The model under review builds one solid part; all positions refer to its coordinate system, in mm. A direction names the side the tool comes from. Coordinates: 2 decimals unless noted, no trailing zeros. Write each loop counter-clockwise with the first axis right and the second up, starting at its lowest first coordinate (ties: lowest second). Pieces come first, ordered by that corner, then holes.
1) Add section B-B, the plane z = 1.25. State the section outline as (x, y) points, then the cut area to 3 significant figures.
2) Add section C-C, the plane x = 3.25. Give the number of separate pieces and of enclosed holes in the cut face, then the cut area to 3 significant figures.
3) Mouldability with a two-part tool opening along X and no side actions: class faces 1 (the flat face through (3, 0, 0)), 2 (the flat face through (-3.458, 1.996, 1.014)), 3 (the cylindrical face through (-5.158, 3.955, 0.887)) as released by +X, released by -X, zero draft, split by the parting line, or undercut.
4) Machinability: for faces 4 (the flat face through (3, 0, 2)), 5 (the flat face through (0.5, 4, 1)), which of the approach directions +Z, -Z, +X, -X, +Y, -Y give a long, thin tool a straight path to every point of the face, cutting with its end or side? Answer none if there is none.
5) For line 1 (Y direction, x = -0.75, z = 0.4); line 2 (X direction, y = -3.75, z = 0.45); line 3 (X direction, y = 3, z = 1.9), list the stretches that pass through material, from the lowest coordinate up.
6) Add section A-A, the plane x = 0. State the section outline as (y, z) points.
7) For P1, Ø0.8, axis at y = -4, z = 1, coming from the +X side; P2, Ø4, axis at x = 1.5, y = -4, coming from the +Z side; P3, Ø0.5, axis at y = 3.5, z = 1, coming from the +X side, all flat-tipped, find the tip position at first contact; note any pin that passes through.
Autodesk Inventor part; units mm, degrees
ref_plane "YZ Plane" through (0, 0, 0) normal (1, 0, 0) x (0, 1, 0)
ref_plane "XZ Plane" through (0, 0, 0) normal (0, 1, 0) x (-1, 0, 0)
ref_plane "XY Plane" through (0, 0, 0) normal (0, 0, 1) x (1, 0, 0)
sketch "スケッチ1" plane through (0, 0, 0) normal (0, 0, 1) x (1, 0, 0)
  circle A0 centre (0, 0) radius 6.5
  arc A1 (2, -1.5) -> (-2, -1.5) centre (0, 0) ccw
  line L0 (2, -1.5) -> (-2, -1.5)
  arc A2 (-2, -1.5) -> (2, -1.5) centre (0, 0) ccw
  dimension "d0" = 13
  dimension "d1" = 5
  dimension "d2" = 4
extrude "押し出し1" add sketch "スケッチ1" along normal blind 2 contours A0 | A2 L0
sketch "スケッチ2" plane through (0, 0, 2) normal (0, 0, 1) x (1, 0, 0)
  circle A0 centre (0, 0) radius 6.5
  line L0 (0.5, -6.5) -> (0, -6.5)
  line L1 (0, -6.5) -> (-0.5, -6.5)
  arc A1 (2, -1.5) -> (-2, -1.5) centre (0, 0) ccw
  arc A2 (3.8971, 2.25) -> (0.5, 4.4721) centre (0, 0) ccw
  arc A3 (3.0311, 1.75) -> (0.5, 3.4641) centre (0, 0) ccw
  arc A4 (-0.5, 4.4721) -> (-3.8971, 2.25) centre (0, 0) ccw
  arc A5 (-0.5, 3.4641) -> (-3.0311, 1.75) centre (0, 0) ccw
  arc A6 (0.5, -3.4641) -> (3.0311, -1.75) centre (0, 0) ccw
  arc A7 (-3.0311, -1.75) -> (-0.5, -3.4641) centre (0, 0) ccw
  arc A8 (-3.8971, -2.25) -> (-0.5, -4.4721) centre (0, 0) ccw
  arc A9 (0.5, -4.4721) -> (3.8971, -2.25) centre (0, 0) ccw
  line L2 (-3.0311, 1.75) -> (-3.8971, 2.25)
  line L3 (-0.5, 3.4641) -> (-0.5, 4.4721)
  line L4 (0.5, 4.4721) -> (0.5, 3.4641)
  line L5 (3.0311, 1.75) -> (3.8971, 2.25)
  line L6 (-3.0311, -1.75) -> (-3.8971, -2.25)
  line L7 (3.0311, -1.75) -> (3.8971, -2.25)
  line L8 (-0.5, -4.4721) -> (-0.5, -3.4641)
  line L9 (0.5, -3.4641) -> (0.5, -4.4721)
extrude "押し出し2" cut sketch "スケッチ2" against normal through all contours L5 A3 L4 A2 | L3 A5 L2 A4 | A6 L7 A9 L9 | A7 L8 A8 L6
chamfer "面取り1" distance 0.2 angle 45 1 edges at (-6.5, 0, 2)
properties part number "SLIPRING_SRG-1-6G_シャフト"
Geometry results:
1. outline: circle Ø13 at (0, 0); hole (-3.9, -2.25) arc R4.5 ccw to (-0.5, -4.47) - (-0.5, -3.46) arc R3.5 cw to (-3.03, -1.75) - close; hole (-3.9, 2.25) - (-3.03, 1.75) arc R3.5 cw to (-0.5, 3.46) - (-0.5, 4.47) arc R4.5 ccw to start; hole (-2, -1.5) - (2, -1.5) arc R2.5 ccw (long way) to start; hole (0.5, -4.47) arc R4.5 ccw to (3.9, -2.25) - (3.03, -1.75) arc R3.5 cw to (0.5, -3.46) - close; hole (0.5, 3.46) arc R3.5 cw to (3.03, 1.75) - (3.9, 2.25) arc R4.5 ccw to (0.5, 4.47) - close
1. area: 101 mm2
2. separate pieces: 3
2. enclosed holes: 0
2. area: 17.5 mm2
3. face 1: zero draft
3. face 2: undercut
3. face 3: split by the parting line
4. face 4: +Z, +X, -X, +Y, -Y
4. face 5: +Z, -Z
5. line 1: y = -6.46 to -4.44, -3.42 to -1.5, 2.38 to 3.42, 4.44 to 6.46
5. line 2: x = -5.31 to -2.49, -0.5 to 0.5, 2.49 to 5.31
5. line 3: x = -5.65 to -3.35, -1.8 to 1.8, 3.35 to 5.65
6. outline: (-6.5, 0) - (-1.5, 0) - (-1.5, 2) - (-6.3, 2) - (-6.5, 1.8) - close; (2.5, 0) - (6.5, 0) - (6.5, 1.8) - (6.3, 2) - (2.5, 2) - close
7. P1: stops at x = 5.41
7. P2: stops at z = 2
7. P3: stops at x = 5.63
